Could you check a few things on this model? Use its own coordinates, in mm. Give positions to 0.01 mm unless a question says otherwise; leave off trailing zeros. Order: outer loops, then holes, each group sorted by start corner. A loop starts at its lowest first (then second) coordinate and runs counter-clockwise, first axis right, second up. Notation, with made-up numbers: (12, 27) -> (36, 27) arc R10 ccw to (36, 46) -> close; hole circle Ø7 at (2, 68.25). An arc over 180 degrees is marked (long way). One line per item, written item: value.
```python
from build123d import *

# Parameters (mm, degrees)
ESBO_O1_W                = 10
ESBO_O1_H                = 15.19
RESSALTO_EXTRUS_O1_DEPTH = 3
CORTE_EXTRUS_O1_DEPTH    = 10
ESBO_O3_R                = 1.8
CORTE_EXTRUS_O2_DEPTH    = 66.535609404
ESBO_O4_R                = 3.5
CORTE_EXTRUS_O3_DEPTH    = 66.535609404
ESBO_O5_R                = 6.5
CORTE_EXTRUS_O4_DEPTH    = 2
FILETE1_R                = 10


with BuildPart() as part:
    # Esboço1 → Ressalto-extrusão1 (new body)
    with BuildSketch(Plane.XY):
        Polygon((-50, -26.19), (50, -26.19), (50, -11), (50, 11), (50, 26.19), (-50, 26.19), align=None)
        with Locations((55, -18.595)):
            Rectangle(ESBO_O1_W, ESBO_O1_H)
        with Locations((55, 18.595)):
            Rectangle(ESBO_O1_W, ESBO_O1_H)
    extrude(amount=RESSALTO_EXTRUS_O1_DEPTH)

    # Esboço2 → Corte-extrusão1 (cut)
    with BuildSketch(Plane(origin=(60, 0, 0), x_dir=(0, 0, -1), z_dir=(1, 0, 0))):
        Polygon((-2, -11), (-2, -12.85), (0, -14.85), (0, -11), align=None)
        Polygon((0, -24.85), (-1.34, -26.19), (0, -26.19), align=None)
        Polygon((0, 11), (0, 14.85), (-2, 12.85), (-2, 11), align=None)
        Polygon((0, 26.19), (0, 24.85), (-1.34, 26.19), align=None)
    extrude(amount=-CORTE_EXTRUS_O1_DEPTH, mode=Mode.SUBTRACT)

    # Esboço3 → Corte-extrusão2 (cut, through all)
    with BuildSketch(Plane(origin=(0, 0, 0), x_dir=(-1, 0, 0), z_dir=(0, 0, -1))):
        with Locations((-55, 19.85)):
            Circle(ESBO_O3_R)
        with Locations(Location((-55, -19.85, 0), (0, 0, 180))):
            Circle(ESBO_O3_R)
    extrude(amount=-CORTE_EXTRUS_O2_DEPTH, mode=Mode.SUBTRACT)

    # Esboço4 → Corte-extrusão3 (cut, through all)
    with BuildSketch(Plane.XY.offset(3)):
        Circle(ESBO_O4_R)
    extrude(amount=-CORTE_EXTRUS_O3_DEPTH, mode=Mode.SUBTRACT)

    # Esboço5 → Corte-extrusão4 (cut)
    with BuildSketch(Plane(origin=(0, 0, 0), x_dir=(-1, 0, 0), z_dir=(0, 0, -1))):
        Circle(ESBO_O5_R)
    extrude(amount=-CORTE_EXTRUS_O4_DEPTH, mode=Mode.SUBTRACT)

    # Filete1
    filete1_edges = [part.edges().sort_by_distance(p)[0] for p in [
        (-50, -26.19, 1.5),
        (-50, 26.19, 1.5),
    ]]
    fillet(filete1_edges, radius=FILETE1_R)


solid = part.part
```
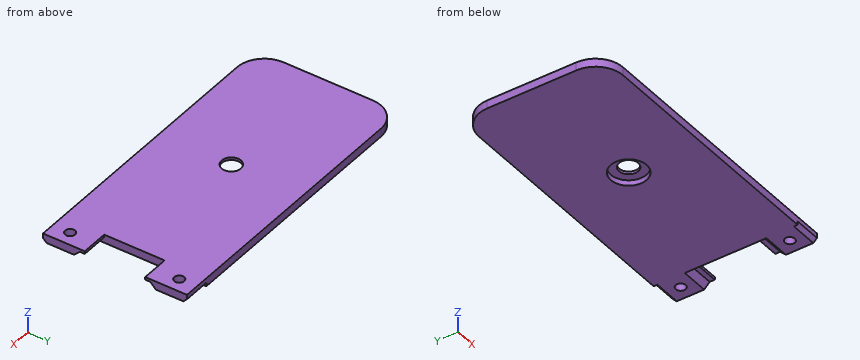
1) Suppose I cut it at C-C, the plane z = 2.5. Write out the boundary of the cut face in (x, y).
Answer below:
outline: (-50, -16.19) arc R10 ccw to (-40, -26.19) -> (60, -26.19) -> (60, -11) -> (50, -11) -> (50, 11) -> (60, 11) -> (60, 26.19) -> (-40, 26.19) arc R10 ccw to (-50, 16.19) -> close; hole circle Ø7 at (0, 0); hole circle Ø3.6 at (55, -19.85); hole circle Ø3.6 at (55, 19.85)
2) If I drill on line 1 along Y through (x, z) = (55, 2.3); line 2 along X through (y, z) = (-10, 1.15); line 3 along Y through (x, z) = (0, 1.45), over which ranges is the centre line in solid material (lowest first)?
Answer below:
line 1: y = -26.19 to -21.65, -18.05 to -11, 11 to 18.05, 21.65 to 26.19
line 2: x = -50 to 50
line 3: y = -26.19 to -6.5, 6.5 to 26.19
3) Suppose I cut it at D-D, the plane y = -19.85. Write out the boundary of the cut face in (x, z).
Answer below:
outline: (-49.31, 0) -> (53.2, 0) -> (53.2, 3) -> (-49.31, 3) -> close; (56.8, 0) -> (60, 0) -> (60, 3) -> (56.8, 3) -> close
4) For P1, Ø6.5, axis at x = 0, y = -2, coming from the -Z side, with a flat end and sliding along its axis, tell me the tip position at first contact or that it passes through.
Answer below:
P1: stops at z = 2
5) Suppose I cut it at B-B, the plane x = 55. Write out the boundary of the cut face in (y, z), then the cut area to 3 significant figures.
Answer below:
outline: (-26.19, 1.34) -> (-24.85, 0) -> (-21.65, 0) -> (-21.65, 3) -> (-26.19, 3) -> close; (-18.05, 0) -> (-14.85, 0) -> (-12.85, 2) -> (-11, 2) -> (-11, 3) -> (-18.05, 3) -> close; (11, 2) -> (12.85, 2) -> (14.85, 0) -> (18.05, 0) -> (18.05, 3) -> (11, 3) -> close; (21.65, 0) -> (24.85, 0) -> (26.19, 1.34) -> (26.19, 3) -> (21.65, 3) -> close
area: 56.3 mm2
6) Suppose I cut it at A-A, the plane x = 0. Write out the boundary of the cut face in (y, z).
Answer below:
outline: (-26.19, 0) -> (-6.5, 0) -> (-6.5, 2) -> (-3.5, 2) -> (-3.5, 3) -> (-26.19, 3) -> close; (3.5, 2) -> (6.5, 2) -> (6.5, 0) -> (26.19, 0) -> (26.19, 3) -> (3.5, 3) -> close
